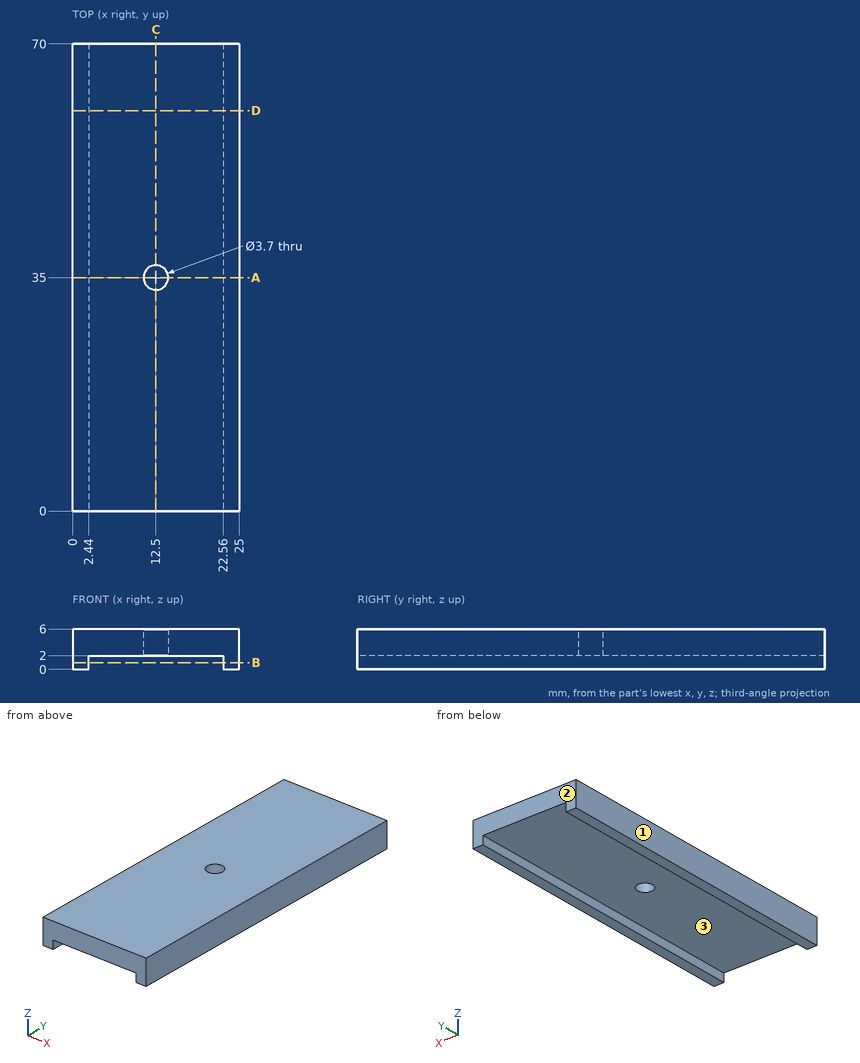
Design review of the part shown in the three views and the two pictorial views. Dimensions are in mm from the part's minimum x, y and z. Round coordinates to 2 decimals unless told otherwise and drop trailing zeros. Loops run counter-clockwise (first coordinate to the right, second up) from the corner with the lowest first, then second, coordinate; pieces in that order, holes last. Notation, with made-up numbers: (30, 60.5) - (62, 60.5) arc R15 ccw to (62, 80.5) - close; hole circle Ø1 at (-26, -5). An arc over 180 degrees is marked (long way). Answer as CSV lines item,"result".
(1) Wall thickness on line 1 (Y direction, x = 12.5, z = 5.1); line 2 (Z direction, x = 2.75, y = 60); line 3 (X direction, y = 37, z = 0.65): over which ranges is each line inside the solid? List them lowest first.
Checked values:
line 1,"y = 0 to 33.15, 36.85 to 70"
line 2,"z = 2 to 6"
line 3,"x = 0 to 2.44, 22.56 to 25"
(2) Mouldability with a two-part tool opening along X and no side actions: class the marked faces 1, 2 and 3 as +X half, -X half, draft (parallel to the pull), parting line (faces both ways), or undercut.
Checked values:
face 1,"-X half"
face 2,"draft"
face 3,"undercut"
(3) Consider section A-A on y = 35. Give the boundary of the cut face in (x, z).
Checked values:
outline,"(0, 0) - (2.44, 0) - (2.44, 2) - (10.65, 2) - (10.65, 6) - (0, 6) - close; (14.35, 2) - (22.56, 2) - (22.56, 0) - (25, 0) - (25, 6) - (14.35, 6) - close"
(4) Insertion check: P1, Ø1.5, axis at x = 10, y = 29, coming from the -Z side; P2, Ø3, axis at x = 12.5, y = 35, coming from the -Z side. Each pin has a flat end and moves straight along its axis. Give the tip position at first contact, or say it passes through.
Checked values:
P1,"stops at z = 2"
P2,"passes through"
(5) Consider section D-D on y = 60. Give the boundary of the cut face in (x, z).
Checked values:
outline,"(0, 0) - (2.44, 0) - (2.44, 2) - (22.56, 2) - (22.56, 0) - (25, 0) - (25, 6) - (0, 6) - close"
(6) Consider section B-B on z = 1. Give the boundary of the cut face in (x, y), then the cut area to 3 significant figures.
Checked values:
outline,"(0, 0) - (2.44, 0) - (2.44, 70) - (0, 70) - close; (22.56, 0) - (25, 0) - (25, 70) - (22.56, 70) - close"
area,"342 mm2"
(7) Consider section C-C on x = 12.5. Give the boundary of the cut face in (y, z).
Checked values:
outline,"(0, 2) - (33.15, 2) - (33.15, 6) - (0, 6) - close; (36.85, 2) - (70, 2) - (70, 6) - (36.85, 6) - close"
